Could you check a few things on this model? Use its own coordinates, in mm. Face numbers are marked on the shaded views. Give positions to 0.01 mm unless a question says otherwise; leave off trailing zeros. Loops run counter-clockwise (first coordinate to the right, second up) from the corner with the lowest first, then second, coordinate; pieces in that order, holes last. Notation, with made-up numbers: (51.5, 70) - (64.5, 70) arc R29 ccw to (64.5, 100) - close; hole circle Ø1 at (51, 60.5). An arc over 180 degrees is marked (long way). One line per item, written item: value. Start each with the question number.
Q1. I'm going to push flat-ended pins straight in: P1, Ø3, axis at x = 40.5, z = 44.5, coming from the -Y side; P2, Ø1.2, axis at x = 35.5, y = -1.5, coming from the -Z side; P3, Ø1.5, axis at x = 100, y = -125.5, coming from the -Z side; P4, Ø6.5, axis at x = 2.5, z = 26.5, coming from the -Y side. Where does each tip first touch, or does it pass through?
Q2. I want a section at B-B (x = 53). Please give me the cut outline in (y, z), then the cut area to 3 significant figures.
Q3. If I drill on line 1 (Y direction, x = 66, z = 4); line 2 (X direction, y = -141.5, z = 20); line 3 (X direction, y = -140, z = 47.5), over which ranges is the centre line in solid material (lowest first)? Write a range as from..to.
Q4. I want a section at A-A (y = -26.5). Please give me the cut outline in (x, z).
Q5. I want a section at D-D (z = 51.5). Count the separate pieces of the cut face and the enclosed holes in it, then the cut area to 3 significant figures.
Q6. I want a section at C-C (x = 84). Please give me the cut outline in (y, z).
Q7. If we mould it in two halves opening along X, with no side actions, what happens to the marked faces 1 and 2? For each: released by +X, released by -X, zero draft, split by the parting line, or undercut.
```python
from build123d import *

# Parameters (mm, degrees)
PAD_DEPTH       = 80
POCKET_DEPTH    = 5
SKETCH002_W     = 33
SKETCH002_H     = 68
POCKET001_DEPTH = 9
SKETCH003_W     = 146.126759
SKETCH003_H     = 66
POCKET002_DEPTH = 5
SKETCH004_W     = 15
SKETCH004_H     = 72
POCKET003_DEPTH = 5
SKETCH005_W     = 20
SKETCH005_H     = 13
POCKET004_DEPTH = 5


with BuildPart() as part:
    # Sketch → Pad (new body)
    with BuildSketch(Plane.XY):
        Polygon((0, 0), (81.5, 0), (81.5, -24), (77.5, -24), (77.5, -4), (6, -4), (6, -39), (128.567111, -141.846018), (136.92335, -131.88744), (130.220486, -148.411324), (0, -40.492439), align=None)
    extrude(amount=PAD_DEPTH)

    # Sketch001 (on Face1 of Pad) → Pocket (cut)
    with BuildSketch(Plane(origin=(0, 0, 0), x_dir=(-1, 0, 0), z_dir=(0, 1, 0))):
        Polygon((-40.75, 35.796221), (-71.1049, 6), (-10.3951, 6), align=None)
        Polygon((-75.5, 69.90665), (-75.5, 10.09335), (-45.0326, 40), align=None)
        Polygon((-71.1049, 74), (-40.75, 44.203779), (-10.3951, 74), align=None)
        Polygon((-6, 69.90665), (-6, 10.09335), (-36.4674, 40), align=None)
    extrude(amount=-POCKET_DEPTH, mode=Mode.SUBTRACT)

    # Sketch002 (on Face22 of Pocket) → Pocket001 (cut)
    with BuildSketch(Plane.YZ.offset(6)):
        with Locations((-21.5, 40)):
            Rectangle(SKETCH002_W, SKETCH002_H)
    extrude(amount=-POCKET001_DEPTH, mode=Mode.SUBTRACT)

    # Sketch003 (on Face18 of Pocket001) → Pocket002 (cut)
    with BuildSketch(Plane(origin=(-19.89418, -24.005342, 0), x_dir=(0.769958, -0.638095, 0), z_dir=(-0.638095, -0.769958, 0))):
        with Locations((106.901389, 40)):
            Rectangle(SKETCH003_W, SKETCH003_H)
    extrude(amount=-POCKET002_DEPTH, mode=Mode.SUBTRACT)

    # Sketch004 (on Face5 of Pocket002) → Pocket003 (cut)
    with BuildSketch(Plane.YZ.offset(81.5)):
        with Locations((-11.5, 40)):
            Rectangle(SKETCH004_W, SKETCH004_H)
    extrude(amount=-POCKET003_DEPTH, mode=Mode.SUBTRACT)

    # Sketch005 (on Face29 of Pocket003) → Pocket004 (cut)
    with BuildSketch(Plane(origin=(163.516532, -66.32999, 0), x_dir=(0.375897, 0.926661, 0), z_dir=(0.926661, -0.375897, 0))):
        with Locations((-72.115176, 40)):
            Rectangle(SKETCH005_W, SKETCH005_H)
    extrude(amount=-POCKET004_DEPTH, mode=Mode.SUBTRACT)


solid = part.part
```
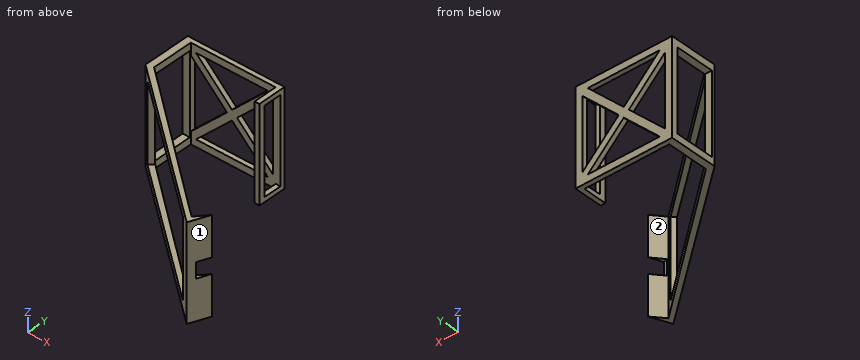
Worked answers:
1. P1: stops at y = -4
1. P2: stops at z = 0
1. P3: passes through
1. P4: stops at y = -45.26
2. outline: (-84.42, 0) - (-78.44, 0) - (-78.44, 7) - (-84.42, 7) - close; (-84.42, 73) - (-78.44, 73) - (-78.44, 80) - (-84.42, 80) - close; (-4, 0) - (0, 0) - (0, 6) - (-4, 6) - close; (-4, 23.77) - (0, 23.77) - (0, 32.18) - (-4, 32.18) - close; (-4, 47.82) - (0, 47.82) - (0, 56.23) - (-4, 56.23) - close; (-4, 74) - (0, 74) - (0, 80) - (-4, 80) - close
2. area: 199 mm²
3. line 1: y = -95.19..-89.35, -4..0
3. line 2: x = 121.88..128.15, 128.86..133.02
3. line 3: x = 120.07..126.37, 130.12..133.63
4. outline: (0, 0) - (6, 0) - (6, 6) - (0, 6) - close; (0, 74) - (6, 74) - (6, 80) - (0, 80) - close
5. separate pieces: 7
5. enclosed holes: 0
5. area: 269 mm²
6. outline: (-110.11, 0) - (-104.45, 0) - (-104.45, 7) - (-110.11, 7) - close; (-110.11, 73) - (-104.45, 73) - (-104.45, 80) - (-110.11, 80) - close
7. face 1: released by +X
7. face 2: undercut
